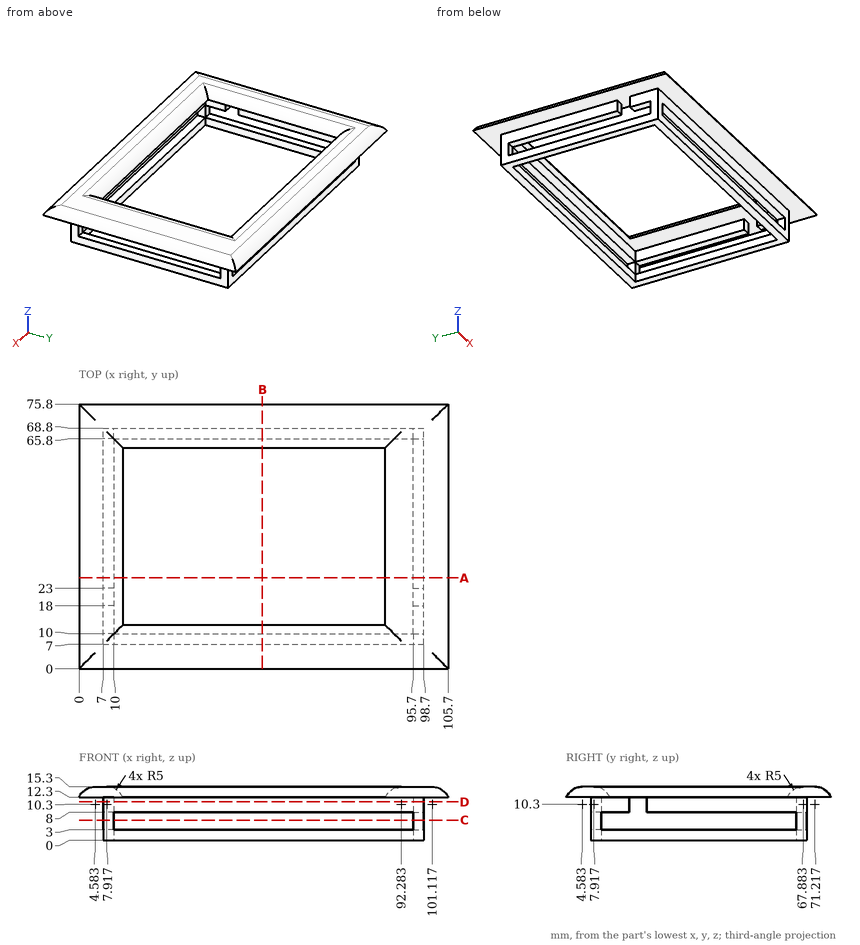
Print and shaded views of the part. All mm, measured from the part's lowest x, y and z. Coordinates: 2 decimals unless noted, no trailing zeros. Write each loop counter-clockwise with the first axis right and the second up, starting at its lowest first coordinate (ties: lowest second). Pieces come first, ordered by that corner, then holes. Notation, with made-up numbers: (38, 16.25) -> (78, 16.25) arc R35 cw to (78, 54.25) -> close; hole circle Ø6 at (13.5, -15.5). An arc over 180 degrees is marked (long way). Use CSV: the item, a comma, the result in double quotes. Start each with the question number.
Q1. Cut at A-A, the plane y = 26. List the corners of the cut face in (x, z).
Q2. Cut at D-D, the plane z = 11. List the corners of the cut face in (x, y).
Q3. Flat gauge pins, fed straight in: pin 1 Ø2 at (x, z) = (33.5, 2.5) entering from -Y; pin 2 Ø2.5 at (x, y) = (98, 48) entering from -Z; pin 3 Ø0.9 at (y, z) = (41.5, 1) entering from +X; pin 4 Ø8 at (x, y) = (86, 26.5) entering from -Z. Where does each tip first touch, or does it go through?
Q4. Drill centre lines: probe 1 along Y at (x, z) = (87.5, 11); probe 2 along X at (y, z) = (50, 10.5); probe 3 along Z at (x, y) = (33.5, 69). Where is each one in solid material? Low to high.
Q5. Cut at C-C, the plane z = 5.75. List the corners of the cut face in (x, y).
Q6. Cut at B-B, the plane x = 52.5. List the corners of the cut face in (y, z).
Checked values:
1,outline,"(0, 12.3) -> (7, 12.3) -> (7, 8) -> (10, 8) -> (10, 12.3) -> (12.5, 12.3) arc R5 ccw to (7.92, 15.3) -> (4.58, 15.3) arc R5 ccw to start; (7, 0) -> (10, 0) -> (10, 3) -> (7, 3) -> close; (87.7, 12.3) -> (95.7, 12.3) -> (95.7, 8) -> (98.7, 8) -> (98.7, 12.3) -> (105.7, 12.3) arc R5 ccw to (101.12, 15.3) -> (92.28, 15.3) arc R5 ccw to start; (95.7, 0) -> (98.7, 0) -> (98.7, 3) -> (95.7, 3) -> close"
2,outline,"(7, 7) -> (98.7, 7) -> (98.7, 18) -> (95.7, 18) -> (95.7, 10) -> (10, 10) -> (10, 18) -> (7, 18) -> close; (7, 23) -> (10, 23) -> (10, 65.8) -> (95.7, 65.8) -> (95.7, 23) -> (98.7, 23) -> (98.7, 68.8) -> (7, 68.8) -> close"
3,pin 1,"stops at y = 7"
3,pin 2,"stops at z = 0"
3,pin 3,"stops at x = 98.7"
3,pin 4,"stops at z = 12.3"
4,probe 1,"y = 7 to 10, 65.8 to 68.8"
4,probe 2,"x = 7 to 10, 95.7 to 98.7"
4,probe 3,"z = 12.3 to 15.3"
5,outline,"(7, 7) -> (10, 7) -> (10, 10) -> (7, 10) -> close; (7, 65.8) -> (10, 65.8) -> (10, 68.8) -> (7, 68.8) -> close; (95.7, 7) -> (98.7, 7) -> (98.7, 10) -> (95.7, 10) -> close; (95.7, 65.8) -> (98.7, 65.8) -> (98.7, 68.8) -> (95.7, 68.8) -> close"
6,outline,"(0, 12.3) -> (7, 12.3) -> (7, 8) -> (10, 8) -> (10, 12.3) -> (12.5, 12.3) arc R5 ccw to (7.92, 15.3) -> (4.58, 15.3) arc R5 ccw to start; (7, 0) -> (10, 0) -> (10, 3) -> (7, 3) -> close; (63.3, 12.3) -> (65.8, 12.3) -> (65.8, 8) -> (68.8, 8) -> (68.8, 12.3) -> (75.8, 12.3) arc R5 ccw to (71.22, 15.3) -> (67.88, 15.3) arc R5 ccw to start; (65.8, 0) -> (68.8, 0) -> (68.8, 3) -> (65.8, 3) -> close"
